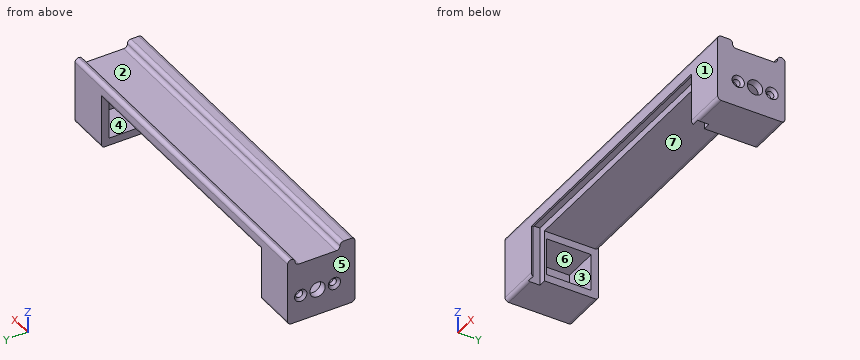
```python
from build123d import *

# Parameters (mm, degrees)
BOSS_EXTRUDE1_DEPTH = 2
SKETCH2_5_W         = 11.5
SKETCH2_5_H         = 14
BOSS_EXTRUDE3_DEPTH = 18
SKETCH3_R           = 2.05
SKETCH3_R_2         = 0.95
CUT_EXTRUDE2_DEPTH  = 96.754895436
CUT_EXTRUDE3_START  = -9.5
SKETCH5_W           = 10.007299984
SKETCH5_H           = 12.005127567
SKETCH5_R           = 0.95
SKETCH5_R_2         = 2.05
CUT_EXTRUDE3_DEPTH  = 9.5
SKETCH6_W           = 10
SKETCH6_H           = 12
SKETCH6_R           = 0.95
SKETCH6_R_2         = 2.05
CUT_EXTRUDE4_DEPTH  = 9.5
CHAMFER1_SIZE       = 0.7
SKETCH11_W          = 2
SKETCH11_H          = 18
BOSS_EXTRUDE6_DEPTH = 93
SKETCH12_W          = 93
SKETCH12_H          = 4
SKETCH12_H_2        = 2
BOSS_EXTRUDE7_DEPTH = 2
SKETCH14_W          = 70
SKETCH14_H          = 14
CUT_EXTRUDE6_DEPTH  = 2
SKETCH16_W          = 70
SKETCH16_H          = 3
CUT_EXTRUDE7_DEPTH  = 2
SKETCH17_W          = 16
SKETCH17_H          = 3
CUT_EXTRUDE8_DEPTH  = 2
SKETCH18_W          = 16
SKETCH18_H          = 3
CUT_EXTRUDE9_DEPTH  = 2
FILLET4_R           = 1


with BuildPart() as part:
    # Sketch2 → Boss-Extrude1 (new body)
    with BuildSketch(Plane(origin=(0, 0, 0), x_dir=(1, 0, 0), z_dir=(0, 1, 0))):
        Polygon((-11.5, 0), (-81.5, 0), (-93, 0), (-93, 14), (-81.5, 14), (-11.5, 14), (0, 14), (0, 0), align=None)
    extrude(amount=BOSS_EXTRUDE1_DEPTH)

    # Sketch2<5> → Boss-Extrude3 (add)
    with BuildSketch(Plane(origin=(0, 0, 0), x_dir=(1, 0, 0), z_dir=(0, 1, 0))):
        with Locations((-87.25, 7)):
            Rectangle(SKETCH2_5_W, SKETCH2_5_H)
        with Locations((-5.75, 7)):
            Rectangle(SKETCH2_5_W, SKETCH2_5_H)
    extrude(amount=BOSS_EXTRUDE3_DEPTH)

    # Sketch3 → Cut-Extrude2 (cut, through all)
    with BuildSketch(Plane.ZY.offset(93)):
        with Locations((-7, 10)):
            Circle(SKETCH3_R)
        with Locations((-7, 14.5)):
            Circle(SKETCH3_R_2)
        with Locations((-7, 5.5)):
            Circle(SKETCH3_R_2)
    extrude(amount=-CUT_EXTRUDE2_DEPTH, mode=Mode.SUBTRACT)

    # Sketch5 → Cut-Extrude3 (cut)
    with BuildSketch(Plane(origin=(-81.5, 0, 0), x_dir=(0, 0, -1), z_dir=(1, 0, 0)).offset(CUT_EXTRUDE3_START)):
        with Locations((6.99901027, 9.998913792)):
            Rectangle(SKETCH5_W, SKETCH5_H)
        with Locations(Location((7, 14.5, 0), (0, 0, 180))):
            Circle(SKETCH5_R, mode=Mode.SUBTRACT)
        with Locations(Location((7, 5.5, 0), (0, 0, 180))):
            Circle(SKETCH5_R, mode=Mode.SUBTRACT)
        with Locations(Location((7, 10, 0), (0, 0, 180))):
            Circle(SKETCH5_R_2, mode=Mode.SUBTRACT)
    extrude(amount=CUT_EXTRUDE3_DEPTH, mode=Mode.SUBTRACT)

    # Sketch6 → Cut-Extrude4 (cut)
    with BuildSketch(Plane.ZY.offset(11.5)):
        with Locations((-7.002660262, 9.996350008)):
            Rectangle(SKETCH6_W, SKETCH6_H)
        with Locations((-7, 14.5)):
            Circle(SKETCH6_R, mode=Mode.SUBTRACT)
        with Locations((-7, 5.5)):
            Circle(SKETCH6_R, mode=Mode.SUBTRACT)
        with Locations((-7, 10)):
            Circle(SKETCH6_R_2, mode=Mode.SUBTRACT)
    extrude(amount=-CUT_EXTRUDE4_DEPTH, mode=Mode.SUBTRACT)

    # Chamfer1
    chamfer1_edges = [part.edges().sort_by_distance(p)[0] for p in [
        (0, 14.5, -7.95),
        (-93, 14.5, -7.95),
        (0, 5.5, -7.95),
        (-93, 5.5, -7.95),
    ]]
    chamfer(chamfer1_edges, length=CHAMFER1_SIZE)

    # Sketch11 → Boss-Extrude6 (add)
    with BuildSketch(Plane(origin=(0, 0, 0), x_dir=(0, 0, -1), z_dir=(1, 0, 0))):
        with Locations((-1, 9)):
            Rectangle(SKETCH11_W, SKETCH11_H)
    extrude(amount=-BOSS_EXTRUDE6_DEPTH)

    # Sketch12 → Boss-Extrude7 (add)
    with BuildSketch(Plane.XY.offset(2)):
        with Locations((-46.5, 2)):
            Rectangle(SKETCH12_W, SKETCH12_H)
        with Locations((-46.5, 17)):
            Rectangle(SKETCH12_W, SKETCH12_H_2)
    extrude(amount=BOSS_EXTRUDE7_DEPTH)

    # Sketch14 → Cut-Extrude6 (cut)
    with BuildSketch(Plane(origin=(0, 2, 0), x_dir=(1, 0, 0), z_dir=(0, 1, 0))):
        with Locations((-46.5, 7)):
            Rectangle(SKETCH14_W, SKETCH14_H)
    extrude(amount=-CUT_EXTRUDE6_DEPTH, mode=Mode.SUBTRACT)

    # Sketch16 → Cut-Extrude7 (cut)
    with BuildSketch(Plane(origin=(0, 0, 0), x_dir=(-1, 0, 0), z_dir=(0, 0, -1))):
        with Locations((46.5, 2)):
            Rectangle(SKETCH16_W, SKETCH16_H)
    extrude(amount=-CUT_EXTRUDE7_DEPTH, mode=Mode.SUBTRACT)

    # Sketch17 → Cut-Extrude8 (cut)
    with BuildSketch(Plane(origin=(-81.5, 0, 0), x_dir=(0, 0, -1), z_dir=(1, 0, 0))):
        with Locations((6, 2)):
            Rectangle(SKETCH17_W, SKETCH17_H)
    extrude(amount=-CUT_EXTRUDE8_DEPTH, mode=Mode.SUBTRACT)

    # Sketch18 → Cut-Extrude9 (cut)
    with BuildSketch(Plane.ZY.offset(11.5)):
        with Locations((-6, 2)):
            Rectangle(SKETCH18_W, SKETCH18_H)
    extrude(amount=-CUT_EXTRUDE9_DEPTH, mode=Mode.SUBTRACT)

    # Fillet4
    fillet4_edges = [part.edges().sort_by_distance(p)[0] for p in [
        (-46.5, 18, 0),
        (-46.5, 4, 2),
        (-46.5, 0, 4),
        (-46.5, 4, 4),
        (-46.5, 16, 2),
        (-46.5, 18, 4),
        (-87.25, 0, -14),
        (-87.25, 18, -14),
        (-5.75, 18, -14),
        (-5.75, 0, -14),
        (-46.5, 16, 4),
    ]]
    fillet(fillet4_edges, radius=FILLET4_R - 0.0001)  # a hair under: the kernel refuses the full size


solid = part.part
```
Can you work these out from the model? Positions are in its coordinate system, mm. Face numbers are marked on the shaded views. A direction names the side the tool comes from. Give positions to 0.01 mm unless a question says otherwise; leave off trailing zeros. Loops run counter-clockwise (first coordinate to the right, second up) from the corner with the lowest first, then second, coordinate; pieces in that order, holes last. Notation, with made-up numbers: M 83.5,36.5 L 113.5,36.5 A24 cw 113.5,70.5 Z; hole C 38.5,-8.75 d5. An arc over 180 degrees is marked long. Use CSV: the item, a comma, the result in double quotes. Start each with the question number.
1. On a 3-axis mill with a long thin cutter (end or side, diameter ignored), from which of +Z, -Z, +X, -X, +Y, -Y can I reach the whole of each face in a straight line? I mean the marked faces 5, 6 and 7. Say none if no direction works.
2. Imagine slicing it at A-A, the plane z = -3.5. Write out the boundary of the cut face in (x, y), plus the area to 3 significant figures.
3. Imagine slicing it at B-B, the plane y = 10. Write out the boundary of the cut face in (x, z), plus the area to 3 significant figures.
4. For P1, Ø3, axis at y = 14.5, z = -7, coming from the -X side; P2, Ø2.5, axis at y = 10, z = -7, coming from the -X side; P3, Ø2.5, axis at y = 5.5, z = -7, coming from the -X side; P4, Ø4, axis at x = -29, y = 12, coming from the +Z side, each with a flat end and sliding along its axis, tell me the tip position at first contact or that it passes through.
5. If we mould it in two halves opening along Z, with no side actions, what happens to the marked faces 1, 2, 3 and 4? For each: released by +Z, released by -Z, zero draft, split by the parting line, or undercut.
6. Imagine slicing it at D-D, the plane z = -7. Count the separate pieces of the cut face and the enclosed holes in it, plus the area to 3 significant figures.
7. If I drill on L1, parallel to Y at x = -1.45, z = -7; L2, parallel to X at y = 7.5, z = -12.25; L3, parallel to X at y = 6.75, z = -3.25, over which ranges is the centre line in solid material (lowest first)?
Response values:
1,face 5,"+Z, -Z, -X, +Y, -Y"
1,face 6,"none"
1,face 7,"-Z, +Y, -Y"
2,outline,"M -93,0 L -81.5,0 L -81.5,0.5 L -83.5,0.5 L -83.5,3.5 L -81.5,3.5 L -81.5,4 L -91,4 L -91,16 L -81.5,16 L -81.5,18 L -93,18 Z; M -11.5,0 L 0,0 L 0,18 L -11.5,18 L -11.5,16 L -2,16 L -2,4 L -11.5,4 L -11.5,3.5 L -9.5,3.5 L -9.5,0.5 L -11.5,0.5 Z"
2,area,"174 mm^2"
3,outline,"M -93,-14 L -81.5,-14 L -81.5,-12 L -91,-12 L -91,-9.05 L -93,-9.05 Z; M -93,-4.95 L -91,-4.95 L -91,-2 L -81.5,-2 L -81.5,0 L -11.5,0 L -11.5,-2 L -2,-2 L -2,-4.95 L 0,-4.95 L 0,2 L -93,2 Z; M -11.5,-14 L 0,-14 L 0,-9.05 L -2,-9.05 L -2,-12 L -11.5,-12 Z"
3,area,"302 mm^2"
4,P1,"x = -92.85"
4,P2,"through"
4,P3,"x = -92.6"
4,P4,"z = 2"
5,face 1,"zero draft"
5,face 2,"released by +Z"
5,face 3,"undercut"
5,face 4,"undercut"
6,separate pieces,"8"
6,enclosed holes,"0"
6,area,"140 mm^2"
7,L1,"0 to 4.55, 6.45 to 7.95, 12.05 to 13.55, 15.45 to 18"
7,L2,"-93 to -81.5, -11.5 to 0"
7,L3,"-93 to -91, -2 to 0"
